```python
from build123d import *

# Parameters (mm, degrees)
SKETCH1_W               = 76.2
SKETCH1_H               = 12.7
BOSS_EXTRUDE1_DEPTH     = 1.016
SKETCH2_R               = 1.524
BOSS_EXTRUDE2_DEPTH     = 12.7
CUT_EXTRUDE1_DEPTH      = 10
CUT_EXTRUDE1_DEPTH_BACK = 11.1600001


with BuildPart() as part:
    # Sketch1 → Boss-Extrude1 (new body)
    with BuildSketch(Plane(origin=(0, 0, 0), x_dir=(1, 0, 0), z_dir=(0, 1, 0))):
        Rectangle(SKETCH1_W, SKETCH1_H)
    extrude(amount=BOSS_EXTRUDE1_DEPTH)

    # Sketch2 → Boss-Extrude2 (add, through all)
    with BuildSketch(Plane(origin=(0, 0, -6.35), x_dir=(-1, 0, 0), z_dir=(0, 0, -1))):
        with BuildLine():
            Line((38.1, 1.016), (38.1, 0))
            Line((38.1, 0), (-38.1, 0))
            add(Edge.make_bspline(
                [(-38.1, 0), (-40.015605578, 0), (-42.822592097, 1.815276702), (-43.811105253, 4.997519765), (-40.168646494, 10.109873022)],
                knots=[0, 0, 0, 0, 0, 1, 1, 1, 1, 1], degree=4))
            ThreePointArc((-40.168646494, 10.109873022), (-35.842209324, 9.799607005), (-38.1, 6.096))
            ThreePointArc((-38.1, 6.096), (-40.64, 3.556), (-38.1, 1.016))
            Line((-38.1, 1.016), (38.1, 1.016))
        make_face()
        with Locations((-38.1, 8.636)):
            Circle(SKETCH2_R, mode=Mode.SUBTRACT)
    extrude(amount=-BOSS_EXTRUDE2_DEPTH)

    # Sketch3 → Cut-Extrude1 (cut, two sides)
    with BuildSketch(Plane.XZ.offset(-1.016)) as cut_extrude1_sk:
        with BuildLine():
            Line((38.1, -6.35), (38.1, -3.947075763))
            Line((38.1, -3.947075763), (37.273899924, -4.092739495))
            add(Edge.make_bspline(
                [(37.273899924, -4.092739495), (34.703704114, -4.800647246), (31.882848561, -6.35), (31.461872823, -6.35)],
                knots=[0.208615082, 0.208615082, 0.208615082, 0.208615082, 1, 1, 1, 1], degree=3))
            Line((31.461872823, -6.35), (38.1, -6.35))
        make_face()
        Polygon((42.354063476, -3.196969595), (39.205663033, -3.752117539), (38.1, -3.947075763), (38.1, -6.35), (42.354063476, -6.35), align=None)
        Polygon((38.1, 3.947075763), (39.205663033, 3.752117539), (42.354063476, 3.196969595), (42.354063476, 6.35), (38.1, 6.35), align=None)
        with BuildLine():
            Line((37.273899924, 4.092739495), (38.1, 3.947075763))
            Line((38.1, 3.947075763), (38.1, 6.35))
            Line((38.1, 6.35), (31.461872823, 6.35))
            add(Edge.make_bspline(
                [(37.273899924, 4.092739495), (34.703704114, 4.800647246), (31.882848561, 6.35), (31.461872823, 6.35)],
                knots=[0.208615082, 0.208615082, 0.208615082, 0.208615082, 1, 1, 1, 1], degree=3))
        make_face()
    extrude(amount=CUT_EXTRUDE1_DEPTH, mode=Mode.SUBTRACT)
    extrude(cut_extrude1_sk.sketch, amount=-CUT_EXTRUDE1_DEPTH_BACK, mode=Mode.SUBTRACT)


solid = part.part
```
Work out the finished part from the listing and answer in its coordinate system (mm). Coordinates: 2 decimals unless noted, no trailing zeros. Loops run counter-clockwise (first coordinate to the right, second up) from the corner with the lowest first, then second, coordinate; pieces in that order, holes last. Notation, with made-up numbers: M -33.5,4 L -10.5,4 A15 cw -10.5,11 Z; hole C 25,14 d4. An arc over 180 degrees is marked long. Use CSV: the item, a comma, the result in double quotes. Start each with the question number.
(1) Given pin 1 Ø5 at (y, z) = (7, 0) entering from -X; pin 2 Ø5 at (x, z) = (-6.5, -3) entering from -Y, each flat-ended and moving along its own axis, determine where each tip first touches the part or whether it passes through.
(2) Consider line 1 (Y direction, x = 38.1, z = 0.25); line 2 (Y direction, x = 35, z = 4.5); line 3 (X direction, y = 9.5, z = 3.25). Determine where each line is inside the solid, lowest interval first.
(3) Find section A-A, the plane x = 5. Give the vertices of the cut face in (y, z).
Recorded:
1,pin 1,"stops at x = 35.56"
1,pin 2,"stops at y = 0"
2,line 1,"y = 0 to 1.02, 6.1 to 7.11, 10.16 to 11.18"
2,line 2,"y = 0 to 1.02"
2,line 3,"x = 35.71 to 36.84, 39.36 to 40.59"
3,outline,"M 0,-6.35 L 1.02,-6.35 L 1.02,6.35 L 0,6.35 Z"
